```python
from build123d import *

# Parameters (mm, degrees)
SKETCH1_W             = 178.5874
SKETCH1_H             = 133.3754
BOSS_EXTRUDE1_DEPTH   = 6.858
FILLET1_R             = 5.08
FILLET2_R             = 5.08
SKETCH3_W             = 101.6
SKETCH3_H             = 83.82
CUT_EXTRUDE2_DEPTH    = 5.08
FILLET4_R             = 0.508
SKETCH5_W             = 45.72
SKETCH5_H             = 17.78
BOSS_EXTRUDE2_DEPTH   = 13.97
SKETCH7_W             = 41.720004
SKETCH7_H             = 13.78
CUT_EXTRUDE3_DEPTH    = 13.97
SKETCH9_W             = 21
SKETCH9_H             = 2.286
CUT_EXTRUDE4_DEPTH    = 2.762
SKETCH10_W            = 28
SKETCH10_H            = 13.97
CUT_EXTRUDE5_DEPTH    = 2.762
SKETCH11_W            = 41.720004
SKETCH11_H            = 13.78
BOSS_EXTRUDE3_DEPTH   = 2.54
MIRROR1_START         = -133.3754
MIRROR1_DEPTH         = 15.78
MIRROR1_2_DEPTH       = 2
MIRROR1_START_2       = -117.5954
MIRROR1_3_OUTLINE_W   = 15.720004
MIRROR1_3_OUTLINE_H   = 13.97
MIRROR1_3_OUTLINE_W_2 = 2
MIRROR1_3_DEPTH       = 2
SKETCH15_W            = 21
SKETCH15_H            = 11.684
CUT_EXTRUDE8_DEPTH    = 2.032
SKETCH17_W            = 20.720004
SKETCH17_H            = 13.97
CUT_EXTRUDE9_DEPTH    = 2.032
SKETCH22_W            = 6.35
SKETCH22_H            = 6.35
CUT_EXTRUDE12_DEPTH   = 7.62
FILLET6_R             = 1.27
FILLET7_R             = 1.27
SKETCH30_W            = 36.1188
SKETCH30_H            = 85.09
CUT_EXTRUDE14_DEPTH   = 5.08
SKETCH31_W            = 3.81
SKETCH31_H            = 5.08
CUT_EXTRUDE15_DEPTH   = 224.866617315
SKETCH32_W            = 3.81
SKETCH32_H            = 5.08
CUT_EXTRUDE16_DEPTH   = 224.866617315
SKETCH33_W            = 6.604
SKETCH33_H            = 6.604
CUT_EXTRUDE17_DEPTH   = 224.866617315


with BuildPart() as part:
    # Sketch1 → Boss-Extrude1 (new body)
    with BuildSketch(Plane(origin=(0, 0, 0), x_dir=(1, 0, 0), z_dir=(0, 1, 0))):
        with Locations((89.2937, 66.6877)):
            Rectangle(SKETCH1_W, SKETCH1_H)
    extrude(amount=BOSS_EXTRUDE1_DEPTH)

    # Fillet1
    fillet1_edges = [part.edges().sort_by_distance(p)[0] for p in [
        (178.5874, 6.858, -66.6877),
    ]]
    fillet(fillet1_edges, radius=FILLET1_R)

    # Fillet2
    fillet2_edges = [part.edges().sort_by_distance(p)[0] for p in [
        (86.7537, 6.858, -133.3754),
        (178.5874, 0.889, -133.3754),
        (177.099502448, 5.370102448, -133.3754),
        (178.5874, 0.889, 0),
        (177.099502448, 5.370102448, 0),
        (0, 6.858, -66.6877),
        (86.7537, 6.858, 0),
    ]]
    fillet(fillet2_edges, radius=FILLET2_R)

    # Sketch3 → Cut-Extrude2 (cut)
    with BuildSketch(Plane(origin=(0, 6.858, 0), x_dir=(1, 0, 0), z_dir=(0, 1, 0))):
        with Locations((66.04, 68.6054)):
            Rectangle(SKETCH3_W, SKETCH3_H)
    extrude(amount=-CUT_EXTRUDE2_DEPTH, mode=Mode.SUBTRACT)

    # Fillet4
    fillet4_edges = [part.edges().sort_by_distance(p)[0] for p in [
        (15.24, 6.858, -68.6054),
        (66.04, 6.858, -26.6954),
        (116.84, 6.858, -68.6054),
        (66.04, 6.858, -110.5154),
    ]]
    fillet(fillet4_edges, radius=FILLET4_R)

    # Sketch5 → Boss-Extrude2 (add)
    with BuildSketch(Plane.XZ):
        with Locations((35.56, -8.89)):
            Rectangle(SKETCH5_W, SKETCH5_H)
    extrude(amount=BOSS_EXTRUDE2_DEPTH)

    # Sketch7 → Cut-Extrude3 (cut)
    with BuildSketch(Plane.XZ.offset(13.97)):
        with Locations((35.559998, -8.89)):
            Rectangle(SKETCH7_W, SKETCH7_H)
    extrude(amount=-CUT_EXTRUDE3_DEPTH, mode=Mode.SUBTRACT)

    # Sketch9 → Cut-Extrude4 (cut)
    with BuildSketch(Plane.XY):
        with Locations((25.199996, -12.827)):
            Rectangle(SKETCH9_W, SKETCH9_H)
    extrude(amount=-CUT_EXTRUDE4_DEPTH, mode=Mode.SUBTRACT)

    # Sketch10 → Cut-Extrude5 (cut)
    with BuildSketch(Plane(origin=(0, 0, -17.78), x_dir=(-1, 0, 0), z_dir=(0, 0, -1))):
        with Locations((-42.420004, -6.985)):
            Rectangle(SKETCH10_W, SKETCH10_H)
    extrude(amount=-CUT_EXTRUDE5_DEPTH, mode=Mode.SUBTRACT)


with BuildPart() as boss_extrude3_tool:
    # Sketch11 → Boss-Extrude3 (new body)
    with BuildSketch(Plane.XZ):
        with Locations((35.559998, -8.89)):
            Rectangle(SKETCH11_W, SKETCH11_H)
    extrude(amount=BOSS_EXTRUDE3_DEPTH)


with BuildPart() as part_1:
    add(part.part)


with BuildPart() as part_2:
    # Boss-Extrude3: joined with boss_extrude3_tool
    add(part_1.part.fuse(boss_extrude3_tool.part, tol=0.00001))

    # Mirror1: read off the stored shape, not the designer's step
    # Mirror1 outline → Mirror1 (add)
    with BuildSketch(Plane.XY.offset(MIRROR1_START)):
        Polygon((12.7, -13.97), (14.699996, -13.97), (14.699996, -2.54), (56.42, -2.54), (56.42, -13.97), (58.42, -13.97), (58.42, 0), (12.7, 0), align=None)
    extrude(amount=MIRROR1_DEPTH)

    # Mirror1 2 outline → Mirror1 2 (add)
    with BuildSketch(Plane.XY.offset(MIRROR1_START)):
        Polygon((14.699996, -2.54), (14.699996, -11.684), (35.699996, -11.684), (35.699996, -13.97), (56.42, -13.97), (56.42, -2.54), align=None)
    extrude(amount=MIRROR1_2_DEPTH)

    # Mirror1 3 outline → Mirror1 3 (add)
    with BuildSketch(Plane.XY.offset(MIRROR1_START_2)):
        with Locations((20.560002, -6.985)):
            Rectangle(MIRROR1_3_OUTLINE_W, MIRROR1_3_OUTLINE_H)
        with Locations((57.42, -6.985)):
            Rectangle(MIRROR1_3_OUTLINE_W_2, MIRROR1_3_OUTLINE_H)
    extrude(amount=MIRROR1_3_DEPTH)

    # Sketch15 → Cut-Extrude8 (cut)
    with BuildSketch(Plane.XY):
        with Locations((25.199996, -5.842)):
            Rectangle(SKETCH15_W, SKETCH15_H)
    cut_extrude8 = extrude(amount=-CUT_EXTRUDE8_DEPTH, mode=Mode.SUBTRACT)

    # Sketch17 → Cut-Extrude9 (cut)
    with BuildSketch(Plane.XY):
        with Locations((46.059998, -6.985)):
            Rectangle(SKETCH17_W, SKETCH17_H)
    cut_extrude9 = extrude(amount=-CUT_EXTRUDE9_DEPTH, mode=Mode.SUBTRACT)

    # Mirror2: Cut-Extrude8, Cut-Extrude9 across plane
    add(cut_extrude8.mirror(Plane(origin=(0, 0, -66.6877), x_dir=(1, 0, 0), z_dir=(0, 0, -1))), mode=Mode.SUBTRACT)
    add(cut_extrude9.mirror(Plane(origin=(0, 0, -66.6877), x_dir=(1, 0, 0), z_dir=(0, 0, -1))), mode=Mode.SUBTRACT)

    # Sketch22 → Cut-Extrude12 (cut)
    with BuildSketch(Plane(origin=(0, 6.858, 0), x_dir=(1, 0, 0), z_dir=(0, 1, 0))):
        with Locations((8.255, 66.6877)):
            Rectangle(SKETCH22_W, SKETCH22_H)
    extrude(amount=-CUT_EXTRUDE12_DEPTH, mode=Mode.SUBTRACT)

    # Fillet6
    fillet6_edges = [part_2.edges().sort_by_distance(p)[0] for p in [
        (58.42, 0, -124.4854),
        (20.560002, 0, -115.5954),
        (12.7, 0, -124.4854),
        (57.42, 0, -115.5954),
    ]]
    fillet(fillet6_edges, radius=FILLET6_R)

    # Fillet7
    fillet7_edges = [part_2.edges().sort_by_distance(p)[0] for p in [
        (57.420002, 0, -17.78),
        (20.560002, 0, -17.78),
        (12.7, 0, -8.89),
        (58.42, 0, -8.89),
    ]]
    fillet(fillet7_edges, radius=FILLET7_R)

    # Sketch30 → Cut-Extrude14 (cut)
    with BuildSketch(Plane(origin=(0, 6.858, 0), x_dir=(1, 0, 0), z_dir=(0, 1, 0))):
        with Locations((150.368, 65.6082)):
            Rectangle(SKETCH30_W, SKETCH30_H)
    extrude(amount=-CUT_EXTRUDE14_DEPTH, mode=Mode.SUBTRACT)

    # Sketch31 → Cut-Extrude15 (cut, through all)
    with BuildSketch(Plane(origin=(0, 6.858, 0), x_dir=(1, 0, 0), z_dir=(0, 1, 0))):
        with Locations((9.525, 125.7554)):
            Rectangle(SKETCH31_W, SKETCH31_H)
    cut_extrude15 = extrude(amount=-CUT_EXTRUDE15_DEPTH, mode=Mode.SUBTRACT)

    # Sketch32 → Cut-Extrude16 (cut, through all)
    with BuildSketch(Plane(origin=(0, 6.858, 0), x_dir=(1, 0, 0), z_dir=(0, 1, 0))):
        with Locations((61.595, 125.7554)):
            Rectangle(SKETCH32_W, SKETCH32_H)
    cut_extrude16 = extrude(amount=-CUT_EXTRUDE16_DEPTH, mode=Mode.SUBTRACT)

    # Mirror3: Cut-Extrude15, Cut-Extrude16 across plane
    add(cut_extrude15.mirror(Plane(origin=(0, 0, -66.6877), x_dir=(1, 0, 0), z_dir=(0, 0, -1))), mode=Mode.SUBTRACT)
    add(cut_extrude16.mirror(Plane(origin=(0, 0, -66.6877), x_dir=(1, 0, 0), z_dir=(0, 0, -1))), mode=Mode.SUBTRACT)

    # Sketch33 → Cut-Extrude17 (cut, through all)
    with BuildSketch(Plane(origin=(0, 6.858, 0), x_dir=(1, 0, 0), z_dir=(0, 1, 0))):
        with Locations((8.382, 117.3734)):
            Rectangle(SKETCH33_W, SKETCH33_H)
    cut_extrude17 = extrude(amount=-CUT_EXTRUDE17_DEPTH, mode=Mode.SUBTRACT)

    # Mirror4: Cut-Extrude17 across plane
    add(cut_extrude17.mirror(Plane(origin=(0, 0, -66.6877), x_dir=(1, 0, 0), z_dir=(0, 0, -1))), mode=Mode.SUBTRACT)


solid = part_2.part
```
Design review of the part built by this model. Coordinates are the model's own, in mm. A direction names the side the tool comes from. Coordinates: 2 decimals unless noted, no trailing zeros. Order: outer loops, then holes, each group sorted by start corner. A loop starts at its lowest first (then second) coordinate and runs counter-clockwise, first axis right, second up.
1) Clearance check with flat-ended pins moving along their axes: pin 1 (1.9 mm diameter, centred on x = 61, y = 5, fed in from +Z); pin 2 (5.5 mm diameter, centred on y = 2.5, z = -9, fed in from -X); pin 3 (1.3 mm diameter, centred on x = 36.5, y = -1.5, fed in from -Z); pin 4 (2 mm diameter, centred on x = 40.5, z = -132, fed in from -Y). State where each tip first meets the part, or that it passes through.
2) Wall thickness on line 1 along Z through (x, y) = (15, -6.75); line 2 along X through (y, z) = (5.5, -30.5); line 3 along X through (y, z) = (-7.5, -127): over which ranges is each line inside the solid? List them lowest first.
3) Mouldability with a two-part tool opening along X and no side actions: class faces 1 (the flat face through (12.7, -8, -9)), 2 (the flat face through (58.42, -8, -9)), 3 (the flat face through (8, 3, -19.304)) as +X half, -X half, draft (parallel to the pull), parting line (faces both ways), or undercut.
4) Take a section at D-D, the plane x = 43. Give the boundary of the cut face in (y, z).
5) For faces 4 (the flat face through (9, 3, -10.16)), 5 (the flat face through (35, -2.54, -125)), 6 (the flat face through (15.24, 4, -68)), list the 3-axis set-ups (+Z, -Z, +X, -X, +Y, -Y) from which the entire face can be reached by the end or side of a thin tool; tool diameter is ignored.
6) Take a section at C-C, the plane z = -43. Give the boundary of the cut face in (x, y), and give its area (3 significant figures).
7) Take a section at B-B, the plane x = 22.5. Give the boundary of the cut face in (y, z).
8) Take a section at A-A, the plane y = -11.25. State how many separate pieces and enclosed holes the cut face has, and give its area (3 significant figures).
Returned:
1. pin 1: stops at z = -0.54
1. pin 2: stops at x = 0
1. pin 3: stops at z = -131.34
1. pin 4: stops at y = -2.54
2. line 1: z = -117.6 to -115.6, -17.78 to -15.78
2. line 2: x = 1.62 to 15.24, 116.84 to 132.31, 168.43 to 176.96
2. line 3: x = 12.7 to 14.7, 56.42 to 58.42
3. face 1: -X half
3. face 2: +X half
3. face 3: undercut
4. outline: (-2.54, -131.34) - (0, -131.34) - (0, -133.38) - (1.78, -133.38) arc R5.08 ccw to (6.86, -128.3) - (6.86, -111.02) arc R0.51 ccw to (6.35, -110.52) - (1.78, -110.52) - (1.78, -26.7) - (6.35, -26.7) arc R0.51 ccw to (6.86, -26.19) - (6.86, -5.08) arc R5.08 ccw to (1.78, 0) - (0, 0) - (0, -2.03) - (-2.54, -2.03) - (-2.54, -15.78) - (0, -15.78) - (0, -117.6) - (-2.54, -117.6) - close
5. face 4: +Y, -Y
5. face 5: -Z, -Y
5. face 6: +Y
6. outline: (0, 0) - (178.59, 0) - (178.59, 1.78) arc R5.08 ccw to (173.51, 6.86) - (168.43, 6.86) - (168.43, 1.78) - (132.31, 1.78) - (132.31, 6.86) - (117.35, 6.86) arc R0.51 ccw to (116.84, 6.35) - (116.84, 1.78) - (15.24, 1.78) - (15.24, 6.35) arc R0.51 ccw to (14.73, 6.86) - (5.08, 6.86) arc R5.08 ccw to (0, 1.78) - close
6. area: 514 mm2
7. outline: (-13.97, -117.6) - (-2.54, -117.6) - (-2.54, -131.34) - (0, -131.34) - (0, -133.38) - (1.78, -133.38) arc R5.08 ccw to (6.86, -128.3) - (6.86, -111.02) arc R0.51 ccw to (6.35, -110.52) - (1.78, -110.52) - (1.78, -26.7) - (6.35, -26.7) arc R0.51 ccw to (6.86, -26.19) - (6.86, -5.08) arc R5.08 ccw to (1.78, 0) - (0, 0) - (0, -2.03) - (-2.54, -2.03) - (-2.54, -15.78) - (-13.97, -15.78) - (-13.97, -17.78) - (-1.27, -17.78) arc R1.27 cw to (0, -19.05) - (0, -114.33) arc R1.27 cw to (-1.27, -115.6) - (-13.97, -115.6) - close
8. separate pieces: 4
8. enclosed holes: 0
8. area: 197 mm2
